Check sheet for the modelled part. Datum: model origin and axes. Units: mm. A direction names the side the tool comes from. Coordinates: 2 decimals unless noted, no trailing zeros. Write each loop counter-clockwise with the first axis right and the second up, starting at its lowest first coordinate (ties: lowest second). Pieces come first, ordered by that corner, then holes. Notation, with made-up numbers: M 83,88 L 107,88 A24 ccw 107,120 Z; hole C 77.25,-40 d6. An arc over 180 degrees is marked long. Answer as CSV lines item,"result". Start each with the question number.
Q1. Mould release check, pull along Z, two halves, no side actions. Record for faces 4 (the flat face through (-12, -3, 9)), 5 (the flat face through (2, -6, 15.25)), 6 (the cylindrical face through (11.6, -1.5, -8.2)): pulls with the +Z half, pulls with the -Z half, needs draft (parallel to the pull), parting line crosses it, or undercut.
Q2. Thickness scan on line 1 along Z through (x, y) = (10, -1.8); line 2 along Z through (x, y) = (-10, -1.6); line 3 along X through (y, z) = (-1.45, -8.25). Record the ranges inside material, lowest first. Write a range as from..to.
Q3. Access from +Z, -Z, +X, -X, +Y, -Y to the whole of each face (thin tool, end or side, straight path). Record for faces 1 (the flat face through (12, -3, -9)), 2 (the flat face through (-2, -6, -15.25)), 3 (the cylindrical face through (-0.54, -10.94, 21.36)).
Q4. Sectioned sample at C-C, the plane y = -10.5. Record the cut outline in (x, z), then the cut area to 3 significant figures.
Q5. Depth check by flat-ended pin: pin 1 Ø1.5 at (x, y) = (-7.5, -8) entering from -Z; pin 2 Ø8 at (x, z) = (5.5, -2.5) entering from +Y; pin 3 Ø8 at (y, z) = (-10, -14) entering from +X; pin 4 Ø1 at (x, y) = (7.5, -3) entering from +Z. Enter the tip coordinate at first touch or a pass-through.
Q6. Sectioned sample at A-A, the plane z = -8.25. Record the cut outline in (x, y).
Q7. Sectioned sample at B-B, the plane x = 0. Record the cut outline in (y, z).
Q8. Sectioned sample at D-D, the plane z = 16.5. Record the cut outline in (x, y).
from build123d import *

# Parameters (mm, degrees)
F1_DEPTH = 17
F2_DEPTH = 3
F3_R     = 2.5
F4_DEPTH = 12.4
F5_DEPTH = 41


with BuildPart() as f1:
    # F0 (on Front) → F1 (new body)
    with BuildSketch(Plane.XZ):
        Polygon((8.5, 15.25), (-8.5, 15.25), (-8.5, 10.912278), (-8.5, 8.306776), (-8.5, 7.193224), (-8.5, 4.587722), (-8.5, -15.25), (8.5, -15.25), (8.5, -11.412278), (8.5, -8.806776), (8.5, -7.693224), (8.5, -5.087722), align=None)
    extrude(amount=F1_DEPTH)

    # F0 (on Front) → F2 (join)
    with BuildSketch(Plane.XZ):
        with BuildLine():
            Line((-8.5, 8.306776), (-8.5, 10.912278))
            ThreePointArc((-8.5, 10.912278), (-13.5, 7.75), (-8.5, 4.587722))
            Line((-8.5, 4.587722), (-8.5, 7.193224))
            ThreePointArc((-8.5, 7.193224), (-11.6, 7.75), (-8.5, 8.306776))
        make_face()
        with BuildLine():
            ThreePointArc((8.5, -11.412278), (13.5, -8.25), (8.5, -5.087722))
            Line((8.5, -5.087722), (8.5, -7.693224))
            ThreePointArc((8.5, -7.693224), (11.6, -8.25), (8.5, -8.806776))
            Line((8.5, -8.806776), (8.5, -11.412278))
        make_face()
    extrude(amount=F2_DEPTH)

    # F3 (on face) → F4 (join)
    with BuildSketch(Plane.XY.offset(15.25)):
        with Locations((0, -8.5)):
            Circle(F3_R)
    extrude(amount=F4_DEPTH)

    # F3 (on face) → F5 (join)
    with BuildSketch(Plane.XY.offset(15.25)):
        with Locations((0, -8.5)):
            Circle(F3_R)
    extrude(amount=-F5_DEPTH)


solid = f1.part
Output:
1,face 4,"needs draft"
1,face 5,"pulls with the +Z half"
1,face 6,"undercut"
2,line 1,"z = -11.75..-9.85, -6.65..-4.75"
2,line 2,"z = 4.25..6.15, 9.35..11.25"
2,line 3,"x = -8.5..8.5, 11.6..13.5"
3,face 1,"+Z, -Z, +X, -Y"
3,face 2,"-Z"
3,face 3,"+Z"
4,outline,"M -8.5,-15.25 L -1.5,-15.25 L -1.5,-25.75 L 1.5,-25.75 L 1.5,-15.25 L 8.5,-15.25 L 8.5,15.25 L 1.5,15.25 L 1.5,27.65 L -1.5,27.65 L -1.5,15.25 L -8.5,15.25 Z"
4,area,"587 mm^2"
5,pin 1,"stops at z = -15.25"
5,pin 2,"stops at y = 0"
5,pin 3,"stops at x = 8.5"
5,pin 4,"stops at z = 15.25"
6,outline,"M -8.5,-17 L 8.5,-17 L 8.5,0 L -8.5,0 Z; M 11.6,-3 L 13.5,-3 L 13.5,0 L 11.6,0 Z"
7,outline,"M -17,-15.25 L -11,-15.25 L -11,-25.75 L -6,-25.75 L -6,-15.25 L 0,-15.25 L 0,15.25 L -6,15.25 L -6,27.65 L -11,27.65 L -11,15.25 L -17,15.25 Z"
8,outline,"C 0,-8.5 d5"
